Study the drawing (mm; zero at the part's minimum x, y, z) and answer. A direction names the side the tool comes from. Coordinates: 2 decimals unless noted, no trailing zeros. Order: outer loops, then holes, each group sorted by start corner. A loop starts at its lowest first (then second) coordinate and runs counter-clockwise, first axis right, second up.
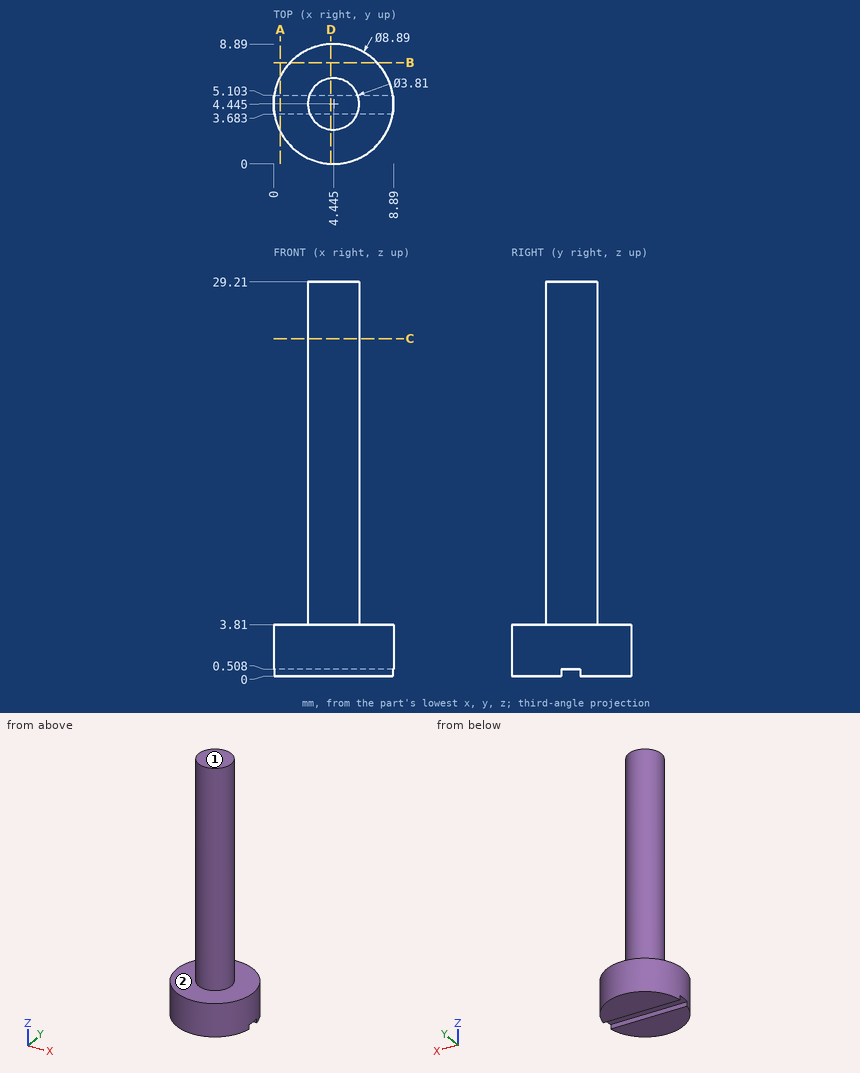
1) Flat-ended cylindrical pins translate along their axes: pin 1 Ø5 at (x, z) = (6.5, 14) entering from +Y; pin 2 Ø0.6 at (x, z) = (5.5, 0.5) entering from +Y (1 decimal); pin 3 Ø1 at (x, z) = (4, 6.5) entering from -Y. Find the tip coordinate at first contact, or state that the pin passes through.
A:
pin 1: stops at y = 6.35
pin 2: stops at y = 8.8
pin 3: stops at y = 2.54
2) A cutting plane is placed at D-D, the plane x = 4.25. Determine the outline of the cut face in (y, z).
A:
outline: (0, 0) - (3.68, 0) - (3.68, 0.51) - (5.1, 0.51) - (5.1, 0) - (8.89, 0) - (8.89, 3.81) - (6.34, 3.81) - (6.34, 29.21) - (2.55, 29.21) - (2.55, 3.81) - (0, 3.81) - close
3) A cutting plane is placed at B-B, the plane y = 7.5. Determine the outline of the cut face in (x, z).
A:
outline: (1.22, 0) - (7.67, 0) - (7.67, 3.81) - (1.22, 3.81) - close
4) Straight lines are drawn through the part: line 1 (Z direction, x = 6.25, y = 2.5); line 2 (Z direction, x = 4, y = 4.5); line 3 (Y direction, x = 4.25, z = 1.75). For each, find the intervals that lie inside material, in ascending order.
A:
line 1: z = 0 to 3.81
line 2: z = 0.51 to 29.21
line 3: y = 0 to 8.89
5) A cutting plane is placed at A-A, the plane x = 0.5. Determine the outline of the cut face in (y, z), and give its area (3 significant figures).
A:
outline: (2.4, 0) - (3.68, 0) - (3.68, 0.51) - (5.1, 0.51) - (5.1, 0) - (6.49, 0) - (6.49, 3.81) - (2.4, 3.81) - close
area: 14.9 mm2
6) Which of the six approach directions +Z, -Z, +X, -X, +Y, -Y give full straight-line access (tool end or side, diameter ignored) to the marked faces 1 and 2?
A:
face 1: +Z, +X, -X, +Y, -Y
face 2: +Z
7) A cutting plane is placed at C-C, the plane z = 25. Determine the outline of the cut face in (x, y) (1 decimal), and give its area (3 significant figures).
A:
outline: circle Ø3.8 at (4.4, 4.4)
area: 11.4 mm2
